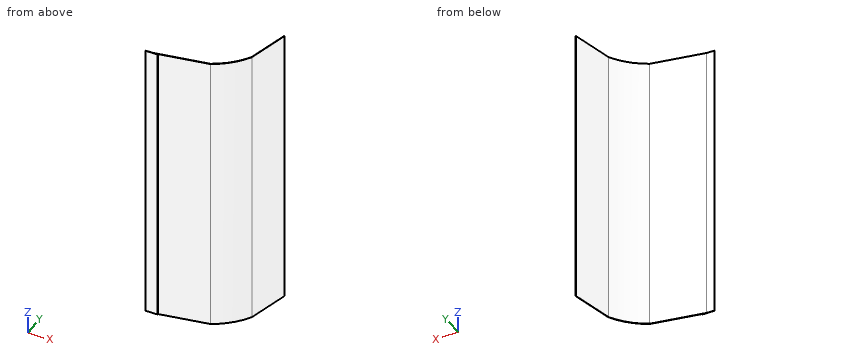
Autodesk Inventor part; units mm, degrees
ref_plane "YZ Plane" through (0, 0, 0) normal (1, 0, 0) x (0, 1, 0)
ref_plane "XZ Plane" through (0, 0, 0) normal (0, 1, 0) x (-1, 0, 0)
ref_plane "XY Plane" through (0, 0, 0) normal (0, 0, 1) x (1, 0, 0)
ref_plane "Work Plane1" through (0, 0, 0) normal (0, 0, 1) x (1, 0, 0)
sketch "Sketch1" plane through (0, 0, 0) normal (0, 0, 1) x (1, 0, 0)
  line L0 (-187.1625, 0.7219) -> (-76.4539, 20.4913)
  line L1 (-17.8884, 75.1531) -> (5.459, 162.2869)
  line L2 (5.459, 162.2869) -> (6.2257, 162.0815)
  line L3 (6.2257, 162.0815) -> (-17.1501, 74.8418)
  line L4 (-76.2, 19.7304) -> (-177.8, 1.5875)
  arc A0 (-76.2, 19.7304) -> (-17.1501, 74.8418) centre (-141.0979, 148.4568) ccw
  arc A1 (-76.4539, 20.4913) -> (-17.8884, 75.1531) centre (-141.0979, 148.4568) ccw
  line L5 (-177.8, 1.5875) -> (-177.8, 0)
  line L6 (-177.8, 0) -> (-203.2, 0)
  line L7 (-203.2, 0) -> (-203.2, 0.3587)
  line L8 (-203.2, 0.3587) -> (-187.1625, 0.7219)
  line L9 (0, 0) -> (0, 25.4) construction
  line L10 (0, 25.4) -> (-44.45, 25.4) construction
  line L11 (-44.45, 25.4) -> (-177.8, 1.5875) construction
  line L12 (-177.8, 1.5875) -> (-177.8, 0) construction
  line L13 (-177.8, 0) -> (0, 0) construction
  dimension "d0" = 0.7937
  dimension "d1" = 0.7937
  dimension "d4" = 76.2
  dimension "d8" = 1.5875
  dimension "d9" = 0
  dimension "d11" = 177.8
  dimension "d12" = 25.4
  dimension "d13" = 44.45
  dimension "d14" = 15
  dimension "d15" = 0.7937
  dimension "d16" = 25.4
extrude "Extrusion1" add sketch "Sketch1" against normal blind 609.6
properties part number "Shovel_Scoop" material "Aluminum-6061"
Here's how the part is built. I have some questions about the finished solid (model axes, mm). Coordinates: 2 decimals unless noted, no trailing zeros. Order: outer loops, then holes, each group sorted by start corner. A loop starts at its lowest first (then second) coordinate and runs counter-clockwise, first axis right, second up. Notation, with made-up numbers: (23.25, -16.5) - (81.25, -16.5) arc R30 cw to (81.25, 21.5) - close; hole circle Ø8 at (44, 15). An arc over 180 degrees is marked (long way). One line per question, with ' | ' between items. Start each with the question number.
1. If we section it at A-A (z = -158): Write out the boundary of the cut face in (x, y), and give its area (3 significant figures).
2. If we section it at B-B (y = 144.5): Write out the boundary of the cut face in (x, z).
3. If we section it at C-C (x = -125): Write out the boundary of the cut face in (y, z), and give its area (3 significant figures).
4. I'm going to push flat-ended pins straight in: pin 1 Ø8 at (x, z) = (-114.5, -490.5) entering from +Y; pin 2 Ø4 at (x, z) = (-94.5, -521) entering from -Y; pin 3 Ø0.5 at (y, z) = (0.5, -410) entering from +X. Where does each tip first touch, or does it pass through?
5. Please list where these lines run through material, in increasing order: line 1 along Y through (x, z) = (-93, -411); line 2 along Y through (x, z) = (-159, -422.5); line 3 along X through (y, z) = (90.5, -84). Write a range as [from, to].
Model answer:
1) outline: (-203.2, 0) - (-177.8, 0) - (-177.8, 1.59) - (-76.2, 19.73) arc R144.16 ccw to (-17.15, 74.84) - (6.23, 162.08) - (5.46, 162.29) - (-17.89, 75.15) arc R143.37 cw to (-76.45, 20.49) - (-187.16, 0.72) - (-203.2, 0.36) - close | area: 241 mm²
2) outline: (0.69, -609.6) - (1.51, -609.6) - (1.51, 0) - (0.69, 0) - close
3) outline: (11.02, -609.6) - (11.82, -609.6) - (11.82, 0) - (11.02, 0) - close | area: 491 mm²
4) pin 1: stops at y = 14.41 | pin 2: stops at y = 16.11 | pin 3: stops at x = -177.8
5) line 1: y = [16.73, 17.54] | line 2: y = [4.94, 5.75] | line 3: x = [-13.78, -12.95]
